Geometry check sheet. Reference: the model listing, model coordinates, mm. A direction names the side the tool comes from. Give positions to 0.01 mm unless a question says otherwise; leave off trailing zeros. One line per question, with ' | ' between items. Start each with the question number.
Q1. Release check for a two-part mould opening along X. For faces 3 (the face through (-20.312, -1.137, 38.546)), 4 (the face through (-18.33, -0.41, 2.25)) record: +X half, -X half, draft (parallel to the pull), parting line (faces both ways), or undercut.
Q2. Thickness scan on L1, parallel to Z at x = -27.5, y = -3; L2, parallel to X at y = 5.5, z = 0; L3, parallel to X at y = 22, z = -2. Record the ranges inside material, lowest first. Write a range as [from, to].
Q3. Set-up check for faces 1 (the face through (-39.15, -0.65, -27.02)), 2 (the face through (2.58, 11.07, 0.19)): record each of +Z, -Z, +X, -X, +Y, -Y from which the full face is reachable in a straight line by a thin tool's end or side.
Q4. Gauge pin test, flat ends, axial feed: P1, Ø2, axis at x = -20.5, y = 11.5, coming from the -Z side; P2, Ø9, axis at x = -25.47, z = 0, coming from the -Y side; P3, Ø1, axis at x = -21, y = -14, coming from the +Z side; P4, Ø6, axis at x = -7, y = 13.5, coming from the +Z side. Record the tip position at first contact, or that the pin passes through.
```python
from build123d import *

# Parameters (mm, degrees)
F2_R          = 7.4871337732
F3_DEPTH      = 38.4
F3_DEPTH_BACK = 28.9757450369


# Not quite as in the source:
# - a fillet or chamfer that OpenCascade refuses, or shapes differently, is made with other operations: its cross-section is extruded or revolved along the edge and cut away or added


with BuildPart() as f1:
    # F0 (on Front) → F1 (revolve)
    with BuildSketch(Plane.XZ):
        Polygon((-10.0024826825, 27.1807126701), (-23.9010660062, 42.7652467351), (-24.3538618088, -43.2729683816), (-10.0024826825, -27.1807126701), (0, -27.1280723152), (4.7837961465, -12.3932333663), (4.7837961465, 0), (4.7837961465, 12.3932333663), (0, 27.1280723152), align=None)
    revolve(axis=Axis((-24.1274639075, 0, -0.2538608233), (-0.005262656, 0, -0.9999861521)))

    # F2 (on Front) → F3 (cut, two sides)
    with BuildSketch(Plane.XZ) as f3_sk:
        with Locations((-25.4709236324, 0)):
            Circle(F2_R)
    extrude(amount=-F3_DEPTH, mode=Mode.SUBTRACT)
    extrude(f3_sk.sketch, amount=F3_DEPTH_BACK, mode=Mode.SUBTRACT)

    # F4: fillet of radius 20 on 1 edges, made by hand

    # F4_s1 → F4_t2 (revolve, cut)
    with BuildSketch(Plane.XZ):
        with BuildLine():
            ThreePointArc((4.2865600872, 13.9247980545), (-1.133885263, 22.4112009628), (-10.0024826825, 27.1807126701))
            Line((-10.0024826825, 27.1807126701), (-9.9078117783, 27.5693480003))
            ThreePointArc((-9.9078117783, 27.5693480003), (-4.9991362788, 27.5543869535), (0.0021050624, 27.5280667761))
            Line((0.0021050624, 27.5280667761), (0.3804517595, 27.2515893532))
            Line((0.3804517595, 27.2515893532), (4.6670118467, 14.0483150925))
            Line((4.6670118467, 14.0483150925), (4.2865600872, 13.9247980545))
        make_face()
    revolve(axis=Axis((-23.9826959839, 0, 27.2542867429), (-0.005262656, 0, -0.9999861521)), mode=Mode.SUBTRACT)


solid = f1.part
```
Working result:
1) face 3: parting line | face 4: undercut
2) L1: z = [-38.31, -7.21], [7.21, 37.61] | L2: x = [-52.51, -32.96], [-17.98, 4.26] | L3: x = [-42.91, -32.69], [-18.26, -5.36]
3) face 1: -Z | face 2: +Z
4) P1: stops at z = -30.7 | P2: passes through | P3: stops at z = 27.42 | P4: stops at z = 25.4
